```python
from build123d import *

# Parameters (mm, degrees)
BOSS_EXTRUDE1_DEPTH      = 0.6
BOSS_EXTRUDE2_DEPTH      = 1.25
BOSS_EXTRUDE2_DEPTH_BACK = 2.1
SKETCH2_R                = 0.725
SKETCH3_R                = 0.5
BOSS_EXTRUDE3_DEPTH      = 1
BOSS_EXTRUDE4_DEPTH      = 1.5


# Read off the part's stored shape, not the designer's step: Boss-Extrude1
with BuildPart() as part:
    # Boss-Extrude1 outline → Boss-Extrude1 (new body)
    with BuildSketch(Plane(origin=(0, 0, 0), x_dir=(1, 0, 0), z_dir=(0, 1, 0))):
        with BuildLine():
            Line((2.459166525, -0.45), (2.030265141, -0.25))
            Line((2.030265141, -0.25), (2.030265141, 0.25))
            Line((2.030265141, 0.25), (2.459166525, 0.45))
            ThreePointArc((2.459166525, 0.45), (2.451963201, 0.487725805), (2.444181164, 0.525336497))
            Line((2.444181164, 0.525336497), (1.971391268, 0.54597895))
            Line((1.971391268, 0.54597895), (1.780049552, 1.007918716))
            Line((1.780049552, 1.007918716), (2.099766075, 1.356828076))
            ThreePointArc((2.099766075, 1.356828076), (2.078674031, 1.388925583), (2.057091378, 1.420695275))
            Line((2.057091378, 1.420695275), (1.612390944, 1.258837554))
            Line((1.612390944, 1.258837554), (1.258837554, 1.612390944))
            Line((1.258837554, 1.612390944), (1.420695275, 2.057091378))
            ThreePointArc((1.420695275, 2.057091378), (1.388925583, 2.078674031), (1.356828076, 2.099766075))
            Line((1.356828076, 2.099766075), (1.007918716, 1.780049552))
            Line((1.007918716, 1.780049552), (0.54597895, 1.971391268))
            Line((0.54597895, 1.971391268), (0.525336497, 2.444181164))
            ThreePointArc((0.525336497, 2.444181164), (0.487725805, 2.451963201), (0.45, 2.459166525))
            Line((0.45, 2.459166525), (0.25, 2.030265141))
            Line((0.25, 2.030265141), (-0.25, 2.030265141))
            Line((-0.25, 2.030265141), (-0.45, 2.459166525))
            ThreePointArc((-0.45, 2.459166525), (-0.487725805, 2.451963201), (-0.525336497, 2.444181164))
            Line((-0.525336497, 2.444181164), (-0.54597895, 1.971391268))
            Line((-0.54597895, 1.971391268), (-1.007918716, 1.780049552))
            Line((-1.007918716, 1.780049552), (-1.356828076, 2.099766075))
            ThreePointArc((-1.356828076, 2.099766075), (-1.388925583, 2.078674031), (-1.420695275, 2.057091378))
            Line((-1.420695275, 2.057091378), (-1.258837554, 1.612390944))
            Line((-1.258837554, 1.612390944), (-1.612390944, 1.258837554))
            Line((-1.612390944, 1.258837554), (-2.057091378, 1.420695275))
            ThreePointArc((-2.057091378, 1.420695275), (-2.078674031, 1.388925583), (-2.099766075, 1.356828076))
            Line((-2.099766075, 1.356828076), (-1.780049552, 1.007918716))
            Line((-1.780049552, 1.007918716), (-1.971391268, 0.54597895))
            Line((-1.971391268, 0.54597895), (-2.444181164, 0.525336497))
            ThreePointArc((-2.444181164, 0.525336497), (-2.451963201, 0.487725805), (-2.459166525, 0.45))
            Line((-2.459166525, 0.45), (-2.030265141, 0.25))
            Line((-2.030265141, 0.25), (-2.030265141, -0.25))
            Line((-2.030265141, -0.25), (-2.459166525, -0.45))
            ThreePointArc((-2.459166525, -0.45), (-2.451963201, -0.487725805), (-2.444181164, -0.525336497))
            Line((-2.444181164, -0.525336497), (-1.971391268, -0.54597895))
            Line((-1.971391268, -0.54597895), (-1.780049552, -1.007918716))
            Line((-1.780049552, -1.007918716), (-2.099766075, -1.356828076))
            ThreePointArc((-2.099766075, -1.356828076), (-2.078674031, -1.388925583), (-2.057091378, -1.420695275))
            Line((-2.057091378, -1.420695275), (-1.612390944, -1.258837554))
            Line((-1.612390944, -1.258837554), (-1.258837554, -1.612390944))
            Line((-1.258837554, -1.612390944), (-1.420695275, -2.057091378))
            ThreePointArc((-1.420695275, -2.057091378), (-1.388925583, -2.078674031), (-1.356828076, -2.099766075))
            Line((-1.356828076, -2.099766075), (-1.007918716, -1.780049552))
            Line((-1.007918716, -1.780049552), (-0.54597895, -1.971391268))
            Line((-0.54597895, -1.971391268), (-0.525336497, -2.444181164))
            ThreePointArc((-0.525336497, -2.444181164), (-0.487725805, -2.451963201), (-0.45, -2.459166525))
            Line((-0.45, -2.459166525), (-0.25, -2.030265141))
            Line((-0.25, -2.030265141), (0.25, -2.030265141))
            Line((0.25, -2.030265141), (0.45, -2.459166525))
            ThreePointArc((0.45, -2.459166525), (0.487725805, -2.451963201), (0.525336497, -2.444181164))
            Line((0.525336497, -2.444181164), (0.54597895, -1.971391268))
            Line((0.54597895, -1.971391268), (1.007918716, -1.780049552))
            Line((1.007918716, -1.780049552), (1.356828076, -2.099766075))
            ThreePointArc((1.356828076, -2.099766075), (1.388925583, -2.078674031), (1.420695275, -2.057091378))
            Line((1.420695275, -2.057091378), (1.258837554, -1.612390944))
            Line((1.258837554, -1.612390944), (1.612390944, -1.258837554))
            Line((1.612390944, -1.258837554), (2.057091378, -1.420695275))
            ThreePointArc((2.057091378, -1.420695275), (2.078674031, -1.388925583), (2.099766075, -1.356828076))
            Line((2.099766075, -1.356828076), (1.780049552, -1.007918716))
            Line((1.780049552, -1.007918716), (1.971391268, -0.54597895))
            Line((1.971391268, -0.54597895), (2.444181164, -0.525336497))
            ThreePointArc((2.444181164, -0.525336497), (2.451963201, -0.487725805), (2.459166525, -0.45))
        make_face()
    extrude(amount=BOSS_EXTRUDE1_DEPTH)

    # Sketch2 → Boss-Extrude2 (add, two sides: drawn at the far end of the back side and taken through both)
    with BuildSketch(Plane(origin=(0, 0.6, 0), x_dir=(1, 0, 0), z_dir=(0, 1, 0)).offset(-BOSS_EXTRUDE2_DEPTH_BACK)):
        with Locations(Location((0, 0, 0), (0, 0, 270))):
            Circle(SKETCH2_R)
    extrude(amount=BOSS_EXTRUDE2_DEPTH + BOSS_EXTRUDE2_DEPTH_BACK)

    # Sketch3 → Boss-Extrude3 (add)
    with BuildSketch(Plane(origin=(0, 1.85, 0), x_dir=(1, 0, 0), z_dir=(0, 1, 0))):
        with Locations(Location((0, 0, 0), (0, 0, 270))):
            Circle(SKETCH3_R)
    extrude(amount=BOSS_EXTRUDE3_DEPTH)

    # Sketch4 → Boss-Extrude4 (add)
    with BuildSketch(Plane(origin=(0, 0, 0), x_dir=(-1, 0, 0), z_dir=(0, -1, 0))):
        with BuildLine():
            Line((0.15, -0.709313048), (0.330979791, -1.022779242))
            ThreePointArc((0.330979791, -1.022779242), (0.367671654, -1.010169567), (0.403884594, -0.996244064))
            Line((0.403884594, -0.996244064), (0.341030972, -0.63978346))
            ThreePointArc((0.341030972, -0.63978346), (0.247964604, -0.68127715), (0.15, -0.709313048))
        make_face()
        with BuildLine():
            ThreePointArc((-0.403884594, -0.996244064), (-0.367671654, -1.010169567), (-0.330979791, -1.022779242))
            Line((-0.330979791, -1.022779242), (-0.15, -0.709313048))
            ThreePointArc((-0.15, -0.709313048), (-0.247964604, -0.68127715), (-0.341030972, -0.63978346))
            Line((-0.341030972, -0.63978346), (-0.403884594, -0.996244064))
        make_face()
        with BuildLine():
            Line((0.570844305, -0.446947177), (0.910975054, -0.570744646))
            ThreePointArc((0.910975054, -0.570744646), (0.930977309, -0.5375), (0.949766889, -0.503555216))
            Line((0.949766889, -0.503555216), (0.672489762, -0.270892081))
            ThreePointArc((0.672489762, -0.270892081), (0.627868418, -0.3625), (0.570844305, -0.446947177))
        make_face()
        with BuildLine():
            ThreePointArc((-0.949766889, -0.503555216), (-0.930977309, -0.5375), (-0.910975054, -0.570744646))
            Line((-0.910975054, -0.570744646), (-0.570844305, -0.446947177))
            ThreePointArc((-0.570844305, -0.446947177), (-0.627868418, -0.3625), (-0.672489762, -0.270892081))
            Line((-0.672489762, -0.270892081), (-0.949766889, -0.503555216))
        make_face()
        with BuildLine():
            ThreePointArc((0.689283119, 0.224752713), (0.713985621, 0.125894929), (0.724584216, 0.024550245))
            Line((0.724584216, 0.024550245), (1.064714965, 0.148347713))
            ThreePointArc((1.064714965, 0.148347713), (1.058668334, 0.186671791), (1.051242702, 0.224752713))
            Line((1.051242702, 0.224752713), (0.689283119, 0.224752713))
        make_face()
        with BuildLine():
            ThreePointArc((-1.051242702, 0.224752713), (-1.058668334, 0.186671791), (-1.064714965, 0.148347713))
            Line((-1.064714965, 0.148347713), (-0.724584216, 0.024550245))
            ThreePointArc((-0.724584216, 0.024550245), (-0.713985621, 0.125894929), (-0.689283119, 0.224752713))
            Line((-0.689283119, 0.224752713), (-1.051242702, 0.224752713))
        make_face()
        with BuildLine():
            ThreePointArc((0.383553243, 0.615233215), (0.466021017, 0.555382221), (0.539283119, 0.484560335))
            Line((0.539283119, 0.484560335), (0.72026291, 0.798026528))
            ThreePointArc((0.72026291, 0.798026528), (0.69099668, 0.823497776), (0.660830371, 0.847896351))
            Line((0.660830371, 0.847896351), (0.383553243, 0.615233215))
        make_face()
        with BuildLine():
            ThreePointArc((-0.660830371, 0.847896351), (-0.69099668, 0.823497776), (-0.72026291, 0.798026528))
            Line((-0.72026291, 0.798026528), (-0.539283119, 0.484560335))
            ThreePointArc((-0.539283119, 0.484560335), (-0.466021017, 0.555382221), (-0.383553243, 0.615233215))
            Line((-0.383553243, 0.615233215), (-0.660830371, 0.847896351))
        make_face()
        with BuildLine():
            ThreePointArc((-0.101645457, 0.717839258), (0, 0.725), (0.101645457, 0.717839258))
            Line((0.101645457, 0.717839258), (0.038791835, 1.074299862))
            ThreePointArc((0.038791835, 1.074299862), (0, 1.075), (-0.038791835, 1.074299862))
            Line((-0.038791835, 1.074299862), (-0.101645457, 0.717839258))
        make_face()
    extrude(amount=BOSS_EXTRUDE4_DEPTH)


solid = part.part
```
The model under review builds one solid part; all positions refer to its coordinate system, in mm. A direction names the side the tool comes from. Give positions to 0.01 mm unless a question says otherwise; leave off trailing zeros. Write each loop counter-clockwise with the first axis right and the second up, starting at its lowest first coordinate (ties: lowest second). Pieces come first, ordered by that corner, then holes.
(1) Tool access review of faces 1 (the flat face through (-1, 0, 1)), 2 (the flat face through (0, -1.5, 0)), 3 (the cylindrical face through (0.032, 1.216, -0.724)): name each direction out of +Z, -Z, +X, -X, +Y, -Y from which nothing blocks a thin tool from reaching the whole face with its end or side.
(2) To check wall thickness, follow L1, parallel to Y at x = 0.5, z = -1.7; L2, parallel to Z at x = 0.05, y = 0.8; L3, parallel to X at y = 2.45, z = -0.05. State the ranges of each line that lie inside material, in increasing order.
(3) Consider section A-A, the plane x = 0.8. Give the boundary of the cut face in (y, z), and give its area (3 significant figures).
(4) Consider section B-B, the plane z = 0.8. Give the boundary of the cut face in (x, y).
(5) Consider section C-C, the plane y = 1.5. Give the boundary of the cut face in (x, z) (3 decimals), and give its area (3 significant figures).
Returned:
1. face 1: -Y
1. face 2: +Z, -Z, +X, -X, -Y
1. face 3: +Y
2. L1: y = 0 to 0.6
2. L2: z = -0.72 to 0.72
2. L3: x = -0.5 to 0.5
3. outline: (-1.5, -0.22) - (0, -0.22) - (0, -1.87) - (0.6, -1.87) - (0.6, 1.87) - (0, 1.87) - (0, 0.53) - (-1.5, 0.53) - (-1.5, 0.38) - (0, 0.38) - (0, -0.05) - (-1.5, -0.05) - close
3. area: 2.73 mm2
4. outline: (-1.87, 0) - (-0.37, 0) - (-0.37, -1.5) - (-0.2, -1.5) - (-0.2, 0) - (0.2, 0) - (0.2, -1.5) - (0.37, -1.5) - (0.37, 0) - (1.87, 0) - (1.87, 0.6) - (-1.87, 0.6) - close
5. outline: circle Ø1.45 at (0, 0)
5. area: 1.65 mm2
